The listing builds one solid part. Answer for the finished solid, in the listing's coordinates (mm). A direction names the side the tool comes from. Give positions to 0.01 mm unless a question says otherwise; leave off trailing zeros. Order: outer loops, then holes, each group sorted by start corner. A loop starts at its lowest first (then second) coordinate and runs counter-clockwise, first axis right, second up. Notation, with made-up numbers: (-13.5, 16) - (21.5, 16) arc R23 ccw to (21.5, 35) - close; hole circle Ø2 at (67.5, 60.5). An arc over 180 degrees is marked (long way). Answer in a Markdown table with one row per item.
from build123d import *

# Parameters (mm, degrees)
BOSS_EXTRUDE1_DEPTH = 3
SKETCH8_R           = 1.5
CUT_EXTRUDE5_DEPTH  = 57.71860365
CUT_EXTRUDE6_DEPTH  = 10


with BuildPart() as part:
    # Sketch1 → Boss-Extrude1 (new body)
    with BuildSketch(Plane(origin=(0, 0, 0), x_dir=(1, 0, 0), z_dir=(0, 1, 0))):
        Polygon((-23, 34), (23, 34), (27, 38), (35, 38), (42, 31), (42, 23), (38, 19), (38, -19), (42, -23), (42, -31), (35, -38), (27, -38), (23, -34), (-23, -34), (-27, -38), (-35, -38), (-42, -31), (-42, -23), (-38, -19), (-38, 19), (-42, 23), (-42, 31), (-35, 38), (-27, 38), align=None)
    extrude(amount=-BOSS_EXTRUDE1_DEPTH)

    # Sketch8 → Cut-Extrude5 (cut, through all)
    with BuildSketch(Plane.XZ.offset(3)):
        with Locations(Location((-29.25, -30, 0), (0, 0, 270))):
            Circle(SKETCH8_R)
        with Locations(Location((29.25, -30, 0), (0, 0, 90))):
            Circle(SKETCH8_R)
        with Locations(Location((29.25, 30, 0), (0, 0, 270))):
            Circle(SKETCH8_R)
        with Locations(Location((-29.25, 30, 0), (0, 0, 90))):
            Circle(SKETCH8_R)
    extrude(amount=-CUT_EXTRUDE5_DEPTH, mode=Mode.SUBTRACT)

    # Sketch11 → Cut-Extrude6 (cut)
    with BuildSketch(Plane.XZ.offset(3)):
        with BuildLine():
            Line((-15, -31), (15, -31))
            ThreePointArc((15, -31), (16, -30), (15, -29))
            Line((15, -29), (-15, -29))
            ThreePointArc((-15, -29), (-16, -30), (-15, -31))
        make_face()
        with BuildLine():
            Line((-15, 31), (15, 31))
            ThreePointArc((15, 31), (16, 30), (15, 29))
            Line((15, 29), (-15, 29))
            ThreePointArc((-15, 29), (-16, 30), (-15, 31))
        make_face()
    extrude(amount=-CUT_EXTRUDE6_DEPTH, mode=Mode.SUBTRACT)


solid = part.part
Item 1: Find section A-A on x = 8. Write down the section's boundary in (y, z), then the cut area to 3 significant figures.
Answer block:
| item | result |
|---|---|
| outline | (-3, -34) - (0, -34) - (0, -31) - (-3, -31) - close; (-3, -29) - (0, -29) - (0, 29) - (-3, 29) - close; (-3, 31) - (0, 31) - (0, 34) - (-3, 34) - close |
| area | 192 mm² |
Item 2: Consider line 1 (Z direction, x = 11.5, y = -2.8); line 2 (X direction, y = -0.8, z = 30); line 3 (X direction, y = -0.7, z = 15.5). Determine where each line is inside the solid, lowest interval first.
Answer block:
| item | result |
|---|---|
| line 1 | -34 to -31, -29 to 29, 31 to 34 |
| line 2 | -42 to -30.75, -27.75 to -16, 16 to 27.75, 30.75 to 42 |
| line 3 | -38 to 38 |
Item 3: Find section D-D on y = -1.6. Count the separate pieces of the cut face and the enclosed holes in it, then the cut area to 3 significant figures.
Answer block:
| item | result |
|---|---|
| separate pieces | 1 |
| enclosed holes | 6 |
| area | 5,400 mm² |
Item 4: Each of these flat-tipped pins is pushed along its axis until it touches: P1, Ø1.5, axis at x = 0.5, y = -2, coming from the +Z side; P2, Ø1.8, axis at x = -29.25, z = 30, coming from the -Y side; P3, Ø0.9, axis at x = -1.5, y = -1, coming from the -Z side; P4, Ø1.5, axis at y = -1, z = -8.5, coming from the +X side. Where does it stop, or does it pass through?
Answer block:
| item | result |
|---|---|
| P1 | z = 34 |
| P2 | through |
| P3 | z = -34 |
| P4 | x = 38 |
Item 5: Find section B-B on z = 30. Write down the section's boundary in (x, y), then the cut area to 3 significant figures.
Answer block:
| item | result |
|---|---|
| outline | (-42, -3) - (-30.75, -3) - (-30.75, 0) - (-42, 0) - close; (-27.75, -3) - (-16, -3) - (-16, 0) - (-27.75, 0) - close; (16, -3) - (27.75, -3) - (27.75, 0) - (16, 0) - close; (30.75, -3) - (42, -3) - (42, 0) - (30.75, 0) - close |
| area | 138 mm² |
Item 6: Determine the mould class of faces 1 (the face through (1, 0, -1)), 2 (the face through (38, -1, 0)), 3 (the face through (-25, -1, -36)) for opening direction X: pulls with the +X half, pulls with the -X half, needs draft (parallel to the pull), parting line crosses it, or undercut.
Answer block:
| item | result |
|---|---|
| face 1 | needs draft |
| face 2 | pulls with the +X half |
| face 3 | undercut |
Item 7: Find section C-C on x = -29.25. Write down the section's boundary in (y, z).
Answer block:
| item | result |
|---|---|
| outline | (-3, -38) - (0, -38) - (0, -31.5) - (-3, -31.5) - close; (-3, -28.5) - (0, -28.5) - (0, 28.5) - (-3, 28.5) - close; (-3, 31.5) - (0, 31.5) - (0, 38) - (-3, 38) - close |
Item 8: Which of the six approach directions +Z, -Z, +X, -X, +Y, -Y give full straight-line access (tool end or side, diameter ignored) to faces 4 (the face through (0, -2, -29)), 5 (the face through (25, -1, 36)), 6 (the face through (25, -1, -36)), 7 (the face through (-38, -1, 0)), 8 (the face through (40, -1, -21))?
Answer block:
| item | result |
|---|---|
| face 4 | +Y, -Y |
| face 5 | +Z, +Y, -Y |
| face 6 | -Z, +Y, -Y |
| face 7 | -X, +Y, -Y |
| face 8 | +X, +Y, -Y |
